from build123d import *

# Parameters (mm, degrees)
BOSS_EXTRUDE1_DEPTH = 23
CUT_EXTRUDE1_START  = -52
CUT_EXTRUDE1_DEPTH  = 52
SKETCH3_W           = 195
SKETCH3_H           = 35
CUT_EXTRUDE2_DEPTH  = 2
FILLET1_R           = 8
CUT_EXTRUDE3_REACH  = 120.528
CHAMFER1_SIZE       = 1
SKETCH16_W          = 28
SKETCH16_H          = 28
SKETCH16_R          = 6
CUT_EXTRUDE4_DEPTH  = 10
SKETCH16_3_R        = 6
CUT_EXTRUDE5_DEPTH  = 126.303631386
CHAMFER2_SIZE       = 2
SKETCH20_W          = 4
SKETCH20_H          = 9


# Read off the part's stored shape, not the designer's step: Cut-Extrude1
with BuildPart() as part:
    # Sketch1 → Boss-Extrude1 (new, symmetric)
    with BuildSketch(Plane.XY):
        Polygon((-104, 0), (104, 0), (99.412073828, 16), (-99.412073828, 16), align=None)
        with BuildLine():
            Line((-54, 68), (-54, 16))
            Line((-54, 16), (54, 16))
            Line((54, 16), (54, 68))
            Line((54, 68), (28, 68))
            Line((28, 68), (28, 52))
            Line((28, 52), (24, 52))
            Line((24, 52), (24, 48))
            ThreePointArc((24, 48), (0, 24), (-24, 48))
            Line((-24, 48), (-24, 52))
            Line((-24, 52), (-28, 52))
            Line((-28, 52), (-28, 68))
            Line((-28, 68), (-54, 68))
        make_face()
    extrude(amount=BOSS_EXTRUDE1_DEPTH, both=True)

    # Cut-Extrude1 outline → Cut-Extrude1 (cut)
    with BuildSketch(Plane(origin=(0, 68, 0), x_dir=(1, 0, 0), z_dir=(0, 1, 0)).offset(CUT_EXTRUDE1_START)):
        with BuildLine():
            ThreePointArc((-54, 0), (-52.698550436, 11.784005345), (-48.856934001, 23))
            Line((-48.856934001, 23), (-54, 23))
            Line((-54, 23), (-54, 0))
        make_face()
        with BuildLine():
            ThreePointArc((-48.856934001, -23), (-52.698550436, -11.784005345), (-54, 0))
            Line((-54, 0), (-54, -23))
            Line((-54, -23), (-48.856934001, -23))
        make_face()
        with BuildLine():
            Line((54, 23), (48.856934001, 23))
            ThreePointArc((48.856934001, 23), (52.698550436, 11.784005345), (54, 0))
            Line((54, 0), (54, 23))
        make_face()
        with BuildLine():
            Line((54, -23), (54, 0))
            ThreePointArc((54, 0), (52.698550436, -11.784005345), (48.856934001, -23))
            Line((48.856934001, -23), (54, -23))
        make_face()
    extrude(amount=CUT_EXTRUDE1_DEPTH, mode=Mode.SUBTRACT)

    # Sketch3 → Cut-Extrude2 (cut)
    with BuildSketch(Plane.XZ):
        Rectangle(SKETCH3_W, SKETCH3_H)
    extrude(amount=-CUT_EXTRUDE2_DEPTH, mode=Mode.SUBTRACT)

    # Fillet1
    fillet1_edges = [part.edges().sort_by_distance(p)[0] for p in [
        (52.698550436, 16, -11.784005345),
        (-52.698550436, 16, -11.784005345),
    ]]
    fillet(fillet1_edges, radius=FILLET1_R)

    # Sketch4 → Cut-Extrude3 (cut, up to next)
    with BuildSketch(Plane(origin=(0, 16, 0), x_dir=(1, 0, 0), z_dir=(0, 1, 0)), mode=Mode.PRIVATE) as cut_extrude3_sk1:
        with BuildLine():
            Line((-85, 6), (-77, 6))
            ThreePointArc((-77, 6), (-71, 0), (-77, -6))
            Line((-77, -6), (-85, -6))
            ThreePointArc((-85, -6), (-91, 0), (-85, 6))
        make_face()
    cut_extrude3_tool1 = extrude(cut_extrude3_sk1.sketch, amount=-CUT_EXTRUDE3_REACH, mode=Mode.PRIVATE) & part.part
    # Sketch4 → Cut-Extrude3 (cut, up to next)
    with BuildSketch(Plane(origin=(0, 16, 0), x_dir=(1, 0, 0), z_dir=(0, 1, 0)), mode=Mode.PRIVATE) as cut_extrude3_sk2:
        with BuildLine():
            Line((85, 6), (77, 6))
            ThreePointArc((77, 6), (71, 0), (77, -6))
            Line((77, -6), (85, -6))
            ThreePointArc((85, -6), (91, 0), (85, 6))
        make_face()
    cut_extrude3_tool2 = extrude(cut_extrude3_sk2.sketch, amount=-CUT_EXTRUDE3_REACH, mode=Mode.PRIVATE) & part.part
    add(cut_extrude3_tool1.solids().sort_by_distance((-81, 16, 0))[0], mode=Mode.SUBTRACT)
    add(cut_extrude3_tool2.solids().sort_by_distance((81, 16, 0))[0], mode=Mode.SUBTRACT)

    # Chamfer1
    chamfer1_edges = [part.edges().sort_by_distance(p)[0] for p in [
        (-91, 16, 0),
        (-81, 16, 6),
        (-71, 16, 0),
        (-81, 16, -6),
        (-81, 2, 6),
        (-91, 2, 0),
        (-81, 2, -6),
        (-71, 2, 0),
        (91, 16, 0),
        (81, 16, -6),
        (71, 16, 0),
        (81, 16, 6),
        (81, 2, -6),
        (91, 2, 0),
        (81, 2, 6),
        (71, 2, 0),
    ]]
    chamfer(chamfer1_edges, length=CHAMFER1_SIZE)

    # Sketch16 → Cut-Extrude4 (cut)
    # profile 1 of 2: a face of its own
    with BuildSketch(Plane.XZ.offset(-2)):
        with Locations((-39, 0)):
            Rectangle(SKETCH16_W, SKETCH16_H)
        with Locations(Location((-39, 0, 0), (0, 0, 270))):
            Circle(SKETCH16_R, mode=Mode.SUBTRACT)
    # profile 2 of 2: a face of its own
    with BuildSketch(Plane.XZ.offset(-2)):
        with Locations((39, 0)):
            Rectangle(SKETCH16_W, SKETCH16_H)
        with Locations(Location((39, 0, 0), (0, 0, 270))):
            Circle(SKETCH16_R, mode=Mode.SUBTRACT)
    extrude(amount=-CUT_EXTRUDE4_DEPTH, mode=Mode.SUBTRACT)

    # Sketch16<3> → Cut-Extrude5 (cut, through all)
    with BuildSketch(Plane.XZ.offset(-2)):
        with Locations(Location((-39, 0, 0), (0, 0, 270))):
            Circle(SKETCH16_3_R)
        with Locations(Location((39, 0, 0), (0, 0, 270))):
            Circle(SKETCH16_3_R)
    extrude(amount=-CUT_EXTRUDE5_DEPTH, mode=Mode.SUBTRACT)

    # Chamfer2
    chamfer2_edges = [part.edges().sort_by_distance(p)[0] for p in [
        (-24, 50, -23),
        (0, 24, -23),
        (24, 50, -23),
        (24, 50, 23),
        (0, 24, 23),
        (-24, 50, 23),
    ]]
    chamfer(chamfer2_edges, length=CHAMFER2_SIZE)

    # Sketch20 → Ø8.0mm Dowel Hole5 (revolve, cut)
    with BuildSketch(Plane(origin=(0, 16, 0), x_dir=(0, 0, -1), z_dir=(1, 0, 0))):
        with Locations((2, 4.5)):
            Rectangle(SKETCH20_W, SKETCH20_H)
    revolve(axis=Axis((0, 9.65, 0), (0, 1, 0)), mode=Mode.SUBTRACT)


solid = part.part
Read the model definition and answer for the solid it produces. Units are mm, in the model's axes. A direction names the side the tool comes from. Coordinates: 2 decimals unless noted, no trailing zeros. Loops run counter-clockwise (first coordinate to the right, second up) from the corner with the lowest first, then second, coordinate; pieces in that order, holes last. Notation, with made-up numbers: (48, 49.25) -> (55, 49.25) arc R28 ccw to (55, 86.25) -> close; hole circle Ø5 at (88.25, 82). An arc over 180 degrees is marked (long way). Write item = value, one per line. Start each with the question number.
1) Find the intervals of material crossed by L1, parallel to X at y = 24, z = 0; L2, parallel to Z at x = 0, y = 19.25; L3, parallel to Y at x = 38.5, z = 13, in increasing order. Write a range as from..to.
2) Given P1, Ø6, axis at x = 20, z = -8, coming from the -Y side; P2, Ø13, axis at y = 62, z = 10, coming from the -X side; P3, Ø11, axis at y = 6, z = -3, coming from the +X side; P4, Ø12, axis at x = -21, y = 49.5, coming from the +Z side, each flat-ended and moving along its own axis, determine where each tip first touches the part or whether it passes through.
3) The mould has two halves that part along X. Classify faces 1 (the face through (25, 7, 0)), 2 (the face through (-1, 19, 23)): pulls with the +X half, pulls with the -X half, needs draft (parallel to the pull), parting line crosses it, or undercut.
4) The part is cut by section A-A, the plane y = 56. Determine the outline of the cut face in (x, z).
5) The part is cut by section C-C, the plane y = 9.5. Determine the outline of the cut face in (x, z), plus the area to 3 significant figures.
6) For faces 3 (the face through (28, 60, 0)), 4 (the face through (32.6, 12, 0.2)), 5 (the face through (-81, 9, 6)), 6 (the face through (91.2, 15.2, 0.1)), determine the directions among +Z, -Z, +X, -X, +Y, -Y from which every point of the face is accessible in a straight line to the end or side of a thin tool.
7) The part is cut by section B-B, the plane x = 80. Determine the outline of the cut face in (y, z).
8) The part is cut by section D-D, the plane x = 0. Determine the outline of the cut face in (y, z).
Result:
q1.L1 = -54..-45, -33..-4, 4..33, 45..54
q1.L2 = -23..-4, 4..23
q1.L3 = 12..68
q2.P1 = 2
q2.P2 = -53.89
q2.P3 = 103.86
q2.P4 = 23
q3.face_1 = undercut
q3.face_2 = needs draft
q4.outline = (-48.86, -23) -> (-28, -23) -> (-28, 23) -> (-48.86, 23) arc R54 ccw to start; (28, -23) -> (48.86, -23) arc R54 ccw to (48.86, 23) -> (28, 23) -> close; hole circle Ø12 at (-39, 0); hole circle Ø12 at (39, 0)
q5.outline = (-101.28, -23) -> (101.28, -23) -> (101.28, 23) -> (-101.28, 23) -> close; hole (-85, -6) -> (-77, -6) arc R6 ccw to (-77, 6) -> (-85, 6) arc R6 ccw to start; hole (-53, -14) -> (-25, -14) -> (-25, 14) -> (-53, 14) -> close; hole (25, -14) -> (53, -14) -> (53, 14) -> (25, 14) -> close; hole (77, -6) -> (85, -6) arc R6 ccw to (85, 6) -> (77, 6) arc R6 ccw to start
q5.area = 7,330 mm²
q6.face_3 = +Z, -Z, +Y
q6.face_4 = -Y
q6.face_5 = +Y, -Y
q6.face_6 = +Y
q7.outline = (0, -23) -> (16, -23) -> (16, -7) -> (15, -6) -> (3, -6) -> (2, -7) -> (2, -17.5) -> (0, -17.5) -> close; (0, 17.5) -> (2, 17.5) -> (2, 7) -> (3, 6) -> (15, 6) -> (16, 7) -> (16, 23) -> (0, 23) -> close
q8.outline = (0, -23) -> (22, -23) -> (24, -21) -> (24, -4) -> (16, -4) -> (16, 4) -> (24, 4) -> (24, 21) -> (22, 23) -> (0, 23) -> (0, 17.5) -> (2, 17.5) -> (2, -17.5) -> (0, -17.5) -> close
